Here's how the part is built. I have some questions about the finished solid (model axes, mm). Round coordinates to 2 decimals unless told otherwise and drop trailing zeros. Write each loop counter-clockwise with the first axis right and the second up, starting at its lowest first coordinate (ties: lowest second). Pieces come first, ordered by that corner, then holes. Notation, with made-up numbers: (65.5, 11) -> (80.5, 11) arc R21 cw to (80.5, 26) -> close; hole circle Ø7 at (27, -20). An arc over 180 degrees is marked (long way). Answer in a Markdown table with one row per item.
from build123d import *

# Parameters (mm, degrees)
BOSS_EXTRUDE1_DEPTH = 10
SKETCH2_R           = 2.5
CUT_EXTRUDE1_DEPTH  = 11


with BuildPart() as part:
    # Sketch1 → Boss-Extrude1 (new body)
    with BuildSketch(Plane.XY):
        with BuildLine():
            Line((-2.297240152, 7.844835842), (-2.388779771, 8.157434107))
            ThreePointArc((-2.388779771, 8.157434107), (-2.74754438, 8.043693174), (-3.100922317, 7.914182256))
            Line((-3.100922317, 7.914182256), (-2.982092925, 7.610905563))
            Line((-2.982092925, 7.610905563), (-3.661072086, 7.308578034))
            Line((-3.661072086, 7.308578034), (-3.806957201, 7.599807686))
            ThreePointArc((-3.806957201, 7.599807686), (-4.139647087, 7.423834723), (-4.464221028, 7.233307031))
            Line((-4.464221028, 7.233307031), (-4.293149129, 6.956121926))
            Line((-4.293149129, 6.956121926), (-4.90723415, 6.537416515))
            Line((-4.90723415, 6.537416515), (-5.102775894, 6.797917194))
            ThreePointArc((-5.102775894, 6.797917194), (-5.398698131, 6.565368115), (-5.684036002, 6.319947367))
            Line((-5.684036002, 6.319947367), (-5.466219987, 6.077762808))
            Line((-5.466219987, 6.077762808), (-5.995673672, 5.55613705))
            Line((-5.995673672, 5.55613705), (-6.234587172, 5.777536049))
            ThreePointArc((-6.234587172, 5.777536049), (-6.484230575, 5.495885174), (-6.721161383, 5.203459394))
            Line((-6.721161383, 5.203459394), (-6.463602037, 5.004059392))
            Line((-6.463602037, 5.004059392), (-6.891407308, 4.396278769))
            Line((-6.891407308, 4.396278769), (-7.166013687, 4.571460142))
            ThreePointArc((-7.166013687, 4.571460142), (-7.361354513, 4.249759962), (-7.542263106, 3.919727955))
            Line((-7.542263106, 3.919727955), (-7.2532386, 3.76952139))
            Line((-7.2532386, 3.76952139), (-7.565645443, 3.095120471))
            Line((-7.565645443, 3.095120471), (-7.867118627, 3.218453745))
            ThreePointArc((-7.867118627, 3.218453745), (-8.00187846, 2.867043968), (-8.120950287, 2.510013234))
            Line((-8.120950287, 2.510013234), (-7.809750106, 2.413827869))
            Line((-7.809750106, 2.413827869), (-7.996717508, 1.694482454))
            Line((-7.996717508, 1.694482454), (-8.315367901, 1.762003596))
            ThreePointArc((-8.315367901, 1.762003596), (-8.385215449, 1.392178821), (-8.438623444, 1.019624623))
            Line((-8.438623444, 1.019624623), (-8.115249818, 0.980551934))
            Line((-8.115249818, 0.980551934), (-8.170768494, 0.239382377))
            Line((-8.170768494, 0.239382377), (-8.496354409, 0.248921202))
            ThreePointArc((-8.496354409, 0.248921202), (-8.499044715, -0.127432098), (-8.4850723, -0.503535563))
            Line((-8.4850723, -0.503535563), (-8.159918723, -0.484239747))
            Line((-8.159918723, -0.484239747), (-8.082204256, -1.223411647))
            Line((-8.082204256, -1.223411647), (-8.404261095, -1.272161724))
            ThreePointArc((-8.404261095, -1.272161724), (-8.33970769, -1.642947245), (-8.258803951, -2.010511701))
            Line((-8.258803951, -2.010511701), (-7.942321126, -1.933467564))
            Line((-7.942321126, -1.933467564), (-7.733871324, -2.646884213))
            Line((-7.733871324, -2.646884213), (-8.042047914, -2.752356326))
            ThreePointArc((-8.042047914, -2.752356326), (-7.912325598, -3.105656715), (-7.767090848, -3.452868339))
            Line((-7.767090848, -3.452868339), (-7.469450794, -3.320552143))
            Line((-7.469450794, -3.320552143), (-7.136965404, -3.985283743))
            Line((-7.136965404, -3.985283743), (-7.421356697, -4.144087931))
            ThreePointArc((-7.421356697, -4.144087931), (-7.230634851, -4.468547824), (-7.025737053, -4.784246948))
            Line((-7.025737053, -4.784246948), (-6.756506167, -4.600911443))
            Line((-6.756506167, -4.600911443), (-6.310671544, -5.195592975))
            Line((-6.310671544, -5.195592975), (-6.562136969, -5.40262514))
            ThreePointArc((-6.562136969, -5.40262514), (-6.316545551, -5.687816128), (-6.05857029, -5.961855923))
            Line((-6.05857029, -5.961855923), (-5.826401873, -5.733393665))
            Line((-5.826401873, -5.733393665), (-5.281547508, -6.238911573))
            Line((-5.281547508, -6.238911573), (-5.492004759, -6.487517532))
            ThreePointArc((-5.492004759, -6.487517532), (-5.199437279, -6.724273342), (-4.896676092, -6.947845943))
            Line((-4.896676092, -6.947845943), (-4.709032228, -6.681599896))
            Line((-4.709032228, -6.681599896), (-4.082670189, -7.08170642))
            Line((-4.082670189, -7.08170642), (-4.245354998, -7.363895772))
            ThreePointArc((-4.245354998, -7.363895772), (-3.915214815, -7.544606879), (-3.577398695, -7.710526478))
            Line((-3.577398695, -7.710526478), (-3.440310413, -7.415054009))
            Line((-3.440310413, -7.415054009), (-2.752572491, -7.696889396))
            Line((-2.752572491, -7.696889396), (-2.862256034, -8.003592343))
            ThreePointArc((-2.862256034, -8.003592343), (-2.505154125, -8.122450542), (-2.143140761, -8.225384348))
            Line((-2.143140761, -8.225384348), (-2.061014191, -7.910182185))
            Line((-2.061014191, -7.910182185), (-1.334004849, -8.064688014))
            Line((-1.334004849, -8.064688014), (-1.387161806, -8.386046871))
            ThreePointArc((-1.387161806, -8.386046871), (-1.014575721, -8.439231962), (-0.64000052, -8.475871597))
            Line((-0.64000052, -8.475871597), (-0.615475277, -8.151070597))
            Line((-0.615475277, -8.151070597), (0.127438807, -8.173280923))
            Line((0.127438807, -8.173280923), (0.132516944, -8.498966952))
            ThreePointArc((0.132516944, -8.498966952), (0.508611982, -8.484769523), (0.883709865, -8.453937359))
            Line((0.883709865, -8.453937359), (0.849845519, -8.129976894))
            Line((0.849845519, -8.129976894), (1.584786475, -8.019177858))
            Line((1.584786475, -8.019177858), (1.64793649, -8.338723243))
            ThreePointArc((1.64793649, -8.338723243), (2.015452477, -8.25759961), (2.379017088, -8.160286619))
            Line((2.379017088, -8.160286619), (2.287851581, -7.847579043))
            Line((2.287851581, -7.847579043), (2.991197802, -7.607331819))
            Line((2.991197802, -7.607331819), (3.110390002, -7.910466107))
            ThreePointArc((3.110390002, -7.910466107), (3.457514671, -7.765023651), (3.797860744, -7.604357552))
            Line((3.797860744, -7.604357552), (3.65232421, -7.312953546))
            Line((3.65232421, -7.312953546), (4.30146957, -6.950979876))
            Line((4.30146957, -6.950979876), (4.47287302, -7.227960082))
            ThreePointArc((4.47287302, -7.227960082), (4.788449499, -7.022873443), (5.09463803, -6.804018176))
            Line((5.09463803, -6.804018176), (4.899408135, -6.543283704))
            Line((4.899408135, -6.543283704), (5.473488567, -6.07121772))
            Line((5.473488567, -6.07121772), (5.691594218, -6.313141473))
            ThreePointArc((5.691594218, -6.313141473), (5.96547962, -6.055002304), (6.227669459, -5.784992058))
            Line((6.227669459, -5.784992058), (5.98902105, -5.56330734))
            Line((5.98902105, -5.56330734), (6.469585137, -4.996321632))
            Line((6.469585137, -4.996321632), (6.727382895, -5.195413302))
            ThreePointArc((6.727382895, -5.195413302), (6.950774318, -4.892518409), (7.160538467, -4.580031535))
            Line((7.160538467, -4.580031535), (6.886141901, -4.4045217))
            Line((6.886141901, -4.4045217), (7.257743919, -3.760839655))
            Line((7.257743919, -3.760839655), (7.546947951, -3.910700273))
            ThreePointArc((7.546947951, -3.910700273), (7.71266541, -3.572784946), (7.863261877, -3.22786503))
            Line((7.863261877, -3.22786503), (7.561936486, -3.10417111))
            Line((7.561936486, -3.10417111), (7.812632839, -2.404481197))
            Line((7.812632839, -2.404481197), (8.12394789, -2.50029412))
            ThreePointArc((8.12394789, -2.50029412), (8.22666509, -2.138219236), (8.31325358, -1.771952288))
            Line((8.31325358, -1.771952288), (7.99468421, -1.704049905))
            Line((7.99468421, -1.704049905), (8.116417311, -0.970840735))
            Line((8.116417311, -0.970840735), (8.439837459, -1.009526456))
            ThreePointArc((8.439837459, -1.009526456), (8.476252984, -0.634929401), (8.496050473, -0.259087541))
            Line((8.496050473, -0.259087541), (8.170476205, -0.249159135))
            Line((8.170476205, -0.249159135), (8.159333453, 0.494003347))
            Line((8.159333453, 0.494003347), (8.484463708, 0.513688219))
            ThreePointArc((8.484463708, 0.513688219), (8.453407134, 0.888767589), (8.405777314, 1.262104493))
            Line((8.405777314, 1.262104493), (8.083662373, 1.213739815))
            Line((8.083662373, 1.213739815), (7.940001904, 1.942969755))
            Line((7.940001904, 1.942969755), (8.256392313, 2.020392532))
            ThreePointArc((8.256392313, 2.020392532), (8.158861823, 2.383898856), (8.045335555, 2.74273145))
            Line((8.045335555, 2.74273145), (7.73703298, 2.637628169))
            Line((7.73703298, 2.637628169), (7.46547216, 3.329487516))
            Line((7.46547216, 3.329487516), (7.762953675, 3.462159766))
            ThreePointArc((7.762953675, 3.462159766), (7.60208398, 3.802409653), (7.426310092, 4.135204762))
            Line((7.426310092, 4.135204762), (7.141728982, 3.976740983))
            Line((7.141728982, 3.976740983), (6.750995999, 4.608992809))
            Line((6.750995999, 4.608992809), (7.020007318, 4.792650337))
            ThreePointArc((7.020007318, 4.792650337), (6.800968902, 5.098707875), (6.568596912, 5.39476919))
            Line((6.568596912, 5.39476919), (6.316883938, 5.18803807))
            Line((6.316883938, 5.18803807), (5.819537272, 5.740361281))
            Line((5.819537272, 5.740361281), (6.051432151, 5.969101182))
            ThreePointArc((6.051432151, 5.969101182), (5.781265088, 6.23112943), (5.499763622, 6.480941297))
            Line((5.499763622, 6.480941297), (5.289009046, 6.232587345))
            Line((5.289009046, 6.232587345), (4.701033829, 6.687229818))
            Line((4.701033829, 6.687229818), (4.888358974, 6.953700205))
            ThreePointArc((4.888358974, 6.953700205), (4.575746658, 7.163277359), (4.254163405, 7.358810619))
            Line((4.254163405, 7.358810619), (4.091141052, 7.076816134))
            Line((4.091141052, 7.076816134), (3.43143529, 7.419165287))
            Line((3.43143529, 7.419165287), (3.568169919, 7.714801581))
            ThreePointArc((3.568169919, 7.714801581), (3.223159965, 7.86519166), (2.871830875, 8.000161712))
            Line((2.871830875, 8.000161712), (2.761780418, 7.693590229))
            Line((2.761780418, 7.693590229), (2.051547597, 7.912642678))
            Line((2.051547597, 7.912642678), (2.133296946, 8.227942886))
            ThreePointArc((2.133296946, 8.227942886), (1.766978258, 8.314312229), (1.397195338, 8.384381026))
            Line((1.397195338, 8.384381026), (1.34365389, 8.063086005))
            Line((1.34365389, 8.063086005), (0.605721477, 8.151801224))
            Line((0.605721477, 8.151801224), (0.629858054, 8.476631337))
            ThreePointArc((0.629858054, 8.476631337), (0.254004417, 8.496203962), (-0.122347206, 8.499119434))
            Line((-0.122347206, 8.499119434), (-0.117658781, 8.173427562))
            Line((-0.117658781, 8.173427562), (-0.85957303, 8.12895417))
            Line((-0.85957303, 8.12895417), (-0.893824994, 8.452873883))
            ThreePointArc((-0.893824994, 8.452873883), (-1.267133336, 8.405020708), (-1.637957411, 8.340689151))
            Line((-1.637957411, 8.340689151), (-1.575189801, 8.021068432))
            Line((-1.575189801, 8.021068432), (-2.297240152, 7.844835842))
        make_face()
    extrude(amount=BOSS_EXTRUDE1_DEPTH)

    # Sketch2 → Cut-Extrude1 (cut, through all)
    with BuildSketch(Plane.XY.offset(10)):
        Circle(SKETCH2_R)
    extrude(amount=-CUT_EXTRUDE1_DEPTH, mode=Mode.SUBTRACT)


solid = part.part
1) For pin 1 (3 mm diameter, centred on x = -6, z = 9, fed in from -Y); pin 2 (3 mm diameter, centred on y = 2.5, z = 8.5, fed in from -X); pin 3 (1.5 mm diameter, centred on x = 3.5, z = 4, fed in from +Y), each with a flat end and sliding along its axis, tell me the tip position at first contact or that it passes through.
Response:
| item | result |
|---|---|
| pin 1 | stops at y = -6.95 |
| pin 2 | stops at x = -8.44 |
| pin 3 | stops at y = 8 |
2) We'd pull the mould along Y, two halves only. Please class faces 1 (the face through (2, -2, 0)), 2 (the face through (-0.54, -2.44, 5.07)): +Y half, -Y half, draft (parallel to the pull), parting line (faces both ways), or undercut.
Response:
| item | result |
|---|---|
| face 1 | draft |
| face 2 | undercut |
3) I want a section at A-A, the plane y = 0. List the corners of the cut face in (x, z) for me.
Response:
| item | result |
|---|---|
| outline | (-8.5, 0) -> (-2.5, 0) -> (-2.5, 10) -> (-8.5, 10) -> close; (2.5, 0) -> (8.17, 0) -> (8.17, 10) -> (2.5, 10) -> close |
4) I need wall thicknesses on line 1 (Y direction, x = 0, z = 7.75); line 2 (Y direction, x = -1, z = 8.5); line 3 (X direction, y = 7.5, z = 1.5). Which ranges of each line are inside material? Lowest first, please. Write a range as [from, to].
Response:
| item | result |
|---|---|
| line 1 | y = [-8.17, -2.5], [2.5, 8.5] |
| line 2 | y = [-8.44, -2.29], [2.29, 8.44] |
| line 3 | x = [-4, -3.76], [-3.23, 3.47] |
